Source: CAD feature listing. Evaluate the final solid. Frame: model axes, mm. Face numbers are marked on the shaded views. A direction names the side the tool comes from. Round coordinates to 2 decimals unless told otherwise and drop trailing zeros. Write each loop counter-clockwise with the first axis right and the second up, starting at its lowest first coordinate (ties: lowest second). Pieces come first, ordered by that corner, then holes. Notation, with made-up numbers: (-4, -14) -> (6, -14) arc R17 cw to (6, 8) -> close; hole circle Ø11 at (47.25, -22.75). An arc over 180 degrees is marked (long way). Put each result on its own line as item: value.
```python
from build123d import *

# Parameters (mm, degrees)
SKETCH2_R          = 6.477
CUT_EXTRUDE1_DEPTH = 30.931960183
SKETCH3_R          = 1.538145308
CUT_EXTRUDE2_DEPTH = 30.931960183


with BuildPart() as part:
    # Sketch1 → Revolve1 (revolve)
    with BuildSketch(Plane.XY):
        Polygon((0, 0), (0, 19.05), (13.0429, 19.05), (13.0429, 12.6365), (5.08, 12.6365), (5.08, 0), align=None)
    revolve(axis=Axis((5.08, 0, 0), (-1, 0, 0)))

    # Sketch2 → Cut-Extrude1 (cut, through all)
    with BuildSketch(Plane.ZY):
        with Locations(Location((0, 0, 0), (0, 0, 270))):
            Circle(SKETCH2_R)
    extrude(amount=-CUT_EXTRUDE1_DEPTH, mode=Mode.SUBTRACT)

    # Sketch3 → Cut-Extrude2 (cut, through all)
    with BuildSketch(Plane.ZY):
        with Locations(Location((0, 16.51, 0), (0, 0, 270))):
            Circle(SKETCH3_R)
        with Locations(Location((14.298079416, 8.255, 0), (0, 0, 270))):
            Circle(SKETCH3_R)
        with Locations(Location((14.298079416, -8.255, 0), (0, 0, 270))):
            Circle(SKETCH3_R)
        with Locations(Location((0, -16.51, 0), (0, 0, 270))):
            Circle(SKETCH3_R)
        with Locations(Location((-14.298079416, -8.255, 0), (0, 0, 270))):
            Circle(SKETCH3_R)
        with Locations(Location((-14.298079416, 8.255, 0), (0, 0, 270))):
            Circle(SKETCH3_R)
    extrude(amount=-CUT_EXTRUDE2_DEPTH, mode=Mode.SUBTRACT)


solid = part.part
```
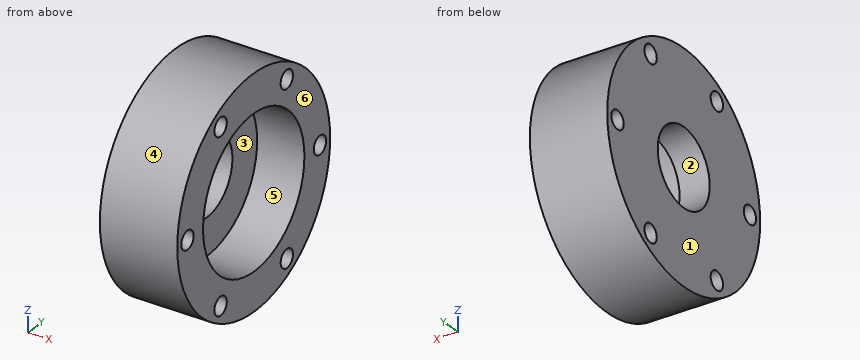
Q1. Cut plane D-D on x = 4.25. Output: boundary loops of the cut face in (y, z) (3 decimals).
Ans:
outline: circle Ø38.1 at (0, 0); hole circle Ø3.076 at (-16.51, 0); hole circle Ø3.076 at (-8.255, -14.298); hole circle Ø3.076 at (-8.255, 14.298); hole circle Ø12.954 at (0, 0); hole circle Ø3.076 at (8.255, -14.298); hole circle Ø3.076 at (8.255, 14.298); hole circle Ø3.076 at (16.51, 0)
Q2. Pin query (flat end, axial travel): pin 1 (1.5 mm diameter, centred on y = -4.5, z = 3, fed in from +X); pin 2 (1 mm diameter, centred on x = 10, z = 11.5, fed in from +Y); pin 3 (6 mm diameter, centred on x = 7.5, y = -13.5, fed in from +Z); pin 4 (2 mm diameter, centred on x = 6.5, y = 14.5, fed in from +Z). Return the tip coordinate at first contact, or that it passes through.
Ans:
pin 1: passes through
pin 2: stops at y = 15.55
pin 3: stops at z = 15.9
pin 4: stops at z = 13.44
Q3. Reachability of the marked faces 5 and 6 from +Z, -Z, +X, -X, +Y, -Y: full face, straight path, thin tool, end or side. Return the list, or none.
Ans:
face 5: +X
face 6: +Z, -Z, +X, +Y, -Y
Q4. Cut plane C-C on y = 8. Output: boundary loops of the cut face in (x, z).
Ans:
outline: (0, -17.29) -> (13.04, -17.29) -> (13.04, -15.81) -> (0, -15.81) -> close; (0, -12.78) -> (13.04, -12.78) -> (13.04, -9.78) -> (5.08, -9.78) -> (5.08, 9.78) -> (13.04, 9.78) -> (13.04, 12.78) -> (0, 12.78) -> close; (0, 15.81) -> (13.04, 15.81) -> (13.04, 17.29) -> (0, 17.29) -> close
Q5. Material intervals for line 1 (Z direction, x = 2.65, y = 0); line 2 (Z direction, x = 9.5, y = -9.5); line 3 (X direction, y = -5.5, z = -10.5), sorted ascending. Write a range as [from, to].
Ans:
line 1: z = [-19.05, -6.48], [6.48, 19.05]
line 2: z = [-16.51, -15.2], [-13.39, -8.33], [8.33, 13.39], [15.2, 16.51]
line 3: x = [0, 5.08]
Q6. Draft query along Z for the marked faces 1, 2, 3 and 4. Return one class per face: +Z half, -Z half, draft (parallel to the pull), parting line (faces both ways), or undercut.
Ans:
face 1: draft
face 2: undercut
face 3: undercut
face 4: parting line
Q7. Cut plane B-B on y = 0. Output: boundary loops of the cut face in (x, z).
Ans:
outline: (0, -19.05) -> (13.04, -19.05) -> (13.04, -12.64) -> (5.08, -12.64) -> (5.08, -6.48) -> (0, -6.48) -> close; (0, 6.48) -> (5.08, 6.48) -> (5.08, 12.64) -> (13.04, 12.64) -> (13.04, 19.05) -> (0, 19.05) -> close
Q8. Cut plane A-A on z = 0. Output: boundary loops of the cut face in (x, y).
Ans:
outline: (0, -19.05) -> (13.04, -19.05) -> (13.04, -18.05) -> (0, -18.05) -> close; (0, -14.97) -> (13.04, -14.97) -> (13.04, -12.64) -> (5.08, -12.64) -> (5.08, -6.48) -> (0, -6.48) -> close; (0, 6.48) -> (5.08, 6.48) -> (5.08, 12.64) -> (13.04, 12.64) -> (13.04, 14.97) -> (0, 14.97) -> close; (0, 18.05) -> (13.04, 18.05) -> (13.04, 19.05) -> (0, 19.05) -> close
